from build123d import *

# Parameters (mm, degrees)
F0_R     = 1.4605
F1_DEPTH = 20.6375


# Not quite as in the source:
# - a length typed as a fraction of an inch, garbled in the dataset ("3 / 203.2 mm" for 3/8 in), is restored


with BuildPart() as f1:
    # F0 (on Top) → F1 (new body, symmetric)
    with BuildSketch(Plane.XY):
        Polygon((-6.35, -6.35), (6.35, -6.35), (3.6661742094, 3.6661742094), (-6.35, 6.35), align=None)
        Circle(F0_R, mode=Mode.SUBTRACT)
    extrude(amount=F1_DEPTH, both=True)


solid = f1.part
Source: CAD feature listing. Evaluate the final solid. Frame: model axes, mm. Give positions to 0.01 mm unless a question says otherwise; leave off trailing zeros. Loops run counter-clockwise (first coordinate to the right, second up) from the corner with the lowest first, then second, coordinate; pieces in that order, holes last. Notation, with made-up numbers: (87.25, 71.5) -> (130.25, 71.5) arc R7 cw to (130.25, 80.5) -> close; hole circle Ø10 at (89.25, -33.75). An arc over 180 degrees is marked (long way). Use a Markdown table: item, result. Add a question column.
1) Line query: line 1 along Y through (x, z) = (0, 2); line 2 along X through (y, z) = (0.5, 15.5); line 3 along X through (y, z) = (-1.25, 17.5). Output: solid intervals per line, ascending. Write a range as [from, to].
2) Section query D-D, the plane x = -3. Return the cut outline in (y, z).
3) Section query C-C, the plane z = 7.5. Return the cut outline in (x, y).
4) Pull-direction query (Y, two-part tool) for faces 1 (the face through (5.027, -1.412, 0.289)), 2 (the face through (-6.35, 0, 0)), 3 (the face through (-0.317, -1.426, -0.289)); classes: +Y half, -Y half, draft (parallel to the pull), parting line (faces both ways), or undercut.
5) Section query B-B, the plane x = -0.5. Return the cut outline in (y, z), then the cut area to 3 significant figures.
6) First-contact query: pin 1 (2 mm diameter, centred on y = -4, z = -2, fed in from +X); pin 2 (6 mm diameter, centred on y = 4.5, z = -3.5, fed in from +X); pin 3 (4 mm diameter, centred on x = 0, y = 0, fed in from +Z); pin 4 (3 mm diameter, centred on x = 4, z = 3.5, fed in from +Y). Flat tips, straight axial feed; report the tip coordinate or a pass-through.
7) Section query A-A, the plane y = 0. Return the cut outline in (x, z).
Numbers:
| question | item | result |
|---|---|---|
| 1 | line 1 | y = [-6.35, -1.46], [1.46, 4.65] |
| 1 | line 2 | x = [-6.35, -1.37], [1.37, 4.51] |
| 1 | line 3 | x = [-6.35, -0.76], [0.76, 4.98] |
| 2 | outline | (-6.35, -20.64) -> (5.45, -20.64) -> (5.45, 20.64) -> (-6.35, 20.64) -> close |
| 3 | outline | (-6.35, -6.35) -> (6.35, -6.35) -> (3.67, 3.67) -> (-6.35, 6.35) -> close; hole circle Ø2.92 at (0, 0) |
| 4 | face 1 | +Y half |
| 4 | face 2 | draft |
| 4 | face 3 | undercut |
| 5 | outline | (-6.35, -20.64) -> (-1.37, -20.64) -> (-1.37, 20.64) -> (-6.35, 20.64) -> close; (1.37, -20.64) -> (4.78, -20.64) -> (4.78, 20.64) -> (1.37, 20.64) -> close |
| 5 | area | 346 mm2 |
| 6 | pin 1 | stops at x = 5.99 |
| 6 | pin 2 | stops at x = 4.25 |
| 6 | pin 3 | stops at z = 20.64 |
| 6 | pin 4 | stops at y = 3.98 |
| 7 | outline | (-6.35, -20.64) -> (-1.46, -20.64) -> (-1.46, 20.64) -> (-6.35, 20.64) -> close; (1.46, -20.64) -> (4.65, -20.64) -> (4.65, 20.64) -> (1.46, 20.64) -> close |
